Part model, mm, in its own coordinate system. A direction names the side the tool comes from. Give positions to 0.01 mm unless a question says otherwise; leave off trailing zeros. Write each loop counter-clockwise with the first axis right and the second up, starting at its lowest first coordinate (ties: lowest second). Pieces come first, ordered by that corner, then holes. Notation, with made-up numbers: (12, 20.5) - (44, 20.5) arc R8 ccw to (44, 26.5) - close; hole circle Ø5 at (73.25, -12). An arc over 180 degrees is marked (long way). Answer in a Markdown table with one row per item. Add a question column.
1. Band-saw the part on B-B on x = -2. Write the cut outline in (y, z).
2. Pull direction Z, two halves, no side cores. Call faces 1 (the flat face through (0, 0, 290)), 2 (the cylindrical face through (11, 2, 262)), 3 (the flat face through (9, 4, 138)): released by +Z, released by -Z, zero draft, split by the parting line, or undercut.
3. Band-saw the part on A-A on z = 105. Write the cut outline in (x, y).
4. Which spindle directions (+Z, -Z, +X, -X, +Y, -Y) get a long thin tool onto all of the face, cutting with end or side? Do faces 4 (the flat face through (13, 0.5, 265)), 5 (the flat face through (16, 1, 147)). Say none if no direction does.
5. Probe line 1 along X through (y, z) = (-1.4, 152); line 2 along Z through (x, y) = (7, 2); line 3 along Z through (x, y) = (6.5, 0.3) (3 decimals). List the from-to ranges inside material, lowest first.
6. Drop flat-ended pins along their axis: pin 1 Ø5.5 at (x, z) = (11, 265) entering from +Y; pin 2 Ø1.8 at (x, z) = (11, 67.5) entering from +Y; pin 3 Ø0.8 at (y, z) = (3.5, 141) entering from -X. Give the stop position or say it passes through.
```python
from build123d import *

# Parameters (mm, degrees)
SKETCH1_W           = 32
SKETCH1_H           = 5
BOSS_EXTRUDE1_DEPTH = 290
SKETCH2_W           = 14
SKETCH2_H           = 280
BOSS_EXTRUDE2_DEPTH = 1.5
SKETCH3_R           = 3
CUT_EXTRUDE1_DEPTH  = 3.5
SKETCH4_R           = 1.75
CUT_EXTRUDE2_DEPTH  = 4
SKETCH5_R           = 0.785
CUT_EXTRUDE3_DEPTH  = 6
SKETCH6_R           = 1.23
CUT_EXTRUDE4_DEPTH  = 7.5
LPATTERN1_COUNT     = 2
LPATTERN1_PITCH     = 95
SKETCH7_R           = 1.23
CUT_EXTRUDE5_DEPTH  = 7.5
SKETCH8_R           = 1.23
CUT_EXTRUDE6_DEPTH  = 7.5
LPATTERN2_COUNT     = 3
LPATTERN2_PITCH     = 61.5
SKETCH9_R           = 1.5
CUT_EXTRUDE7_DEPTH  = 7.5
SKETCH10_R          = 0.785
CUT_EXTRUDE8_DEPTH  = 8


with BuildPart() as part:
    # Sketch1 → Boss-Extrude1 (new body)
    with BuildSketch(Plane.XY):
        Rectangle(SKETCH1_W, SKETCH1_H)
    extrude(amount=BOSS_EXTRUDE1_DEPTH)

    # Sketch2 → Boss-Extrude2 (add)
    with BuildSketch(Plane(origin=(0, 2.5, 0), x_dir=(1, 0, 0), z_dir=(0, 1, 0))):
        with Locations((9, -140)):
            Rectangle(SKETCH2_W, SKETCH2_H)
    extrude(amount=BOSS_EXTRUDE2_DEPTH)

    # Sketch3 → Cut-Extrude1 (cut)
    with BuildSketch(Plane(origin=(0, 4, 0), x_dir=(1, 0, 0), z_dir=(0, 1, 0))):
        with Locations((11, -10)):
            Circle(SKETCH3_R)
        with Locations((11, -145)):
            Circle(SKETCH3_R)
        with Locations((11, -265)):
            Circle(SKETCH3_R)
    extrude(amount=-CUT_EXTRUDE1_DEPTH, mode=Mode.SUBTRACT)

    # Sketch4 → Cut-Extrude2 (cut, through all)
    with BuildSketch(Plane(origin=(0, 0.5, 0), x_dir=(1, 0, 0), z_dir=(0, 1, 0))):
        with Locations((11, -10)):
            Circle(SKETCH4_R)
        with Locations((11, -145)):
            Circle(SKETCH4_R)
        with Locations((11, -265)):
            Circle(SKETCH4_R)
    extrude(amount=-CUT_EXTRUDE2_DEPTH, mode=Mode.SUBTRACT)

    # Sketch5 → Cut-Extrude3 (cut, through all)
    with BuildSketch(Plane(origin=(0, 2.5, 0), x_dir=(1, 0, 0), z_dir=(0, 1, 0))):
        with Locations((-11.5, -282.5)):
            Circle(SKETCH5_R)
        with Locations((6.5, -282.5)):
            Circle(SKETCH5_R)
        with Locations((-11.5, -287.5)):
            Circle(SKETCH5_R)
        with Locations((6.5, -287.5)):
            Circle(SKETCH5_R)
    extrude(amount=-CUT_EXTRUDE3_DEPTH, mode=Mode.SUBTRACT)

    # Sketch6 → Cut-Extrude4 (cut, through all)
    with BuildSketch(Plane(origin=(0, 4, 0), x_dir=(1, 0, 0), z_dir=(0, 1, 0))):
        with Locations((11, -20)):
            Circle(SKETCH6_R)
    cut_extrude4 = extrude(amount=-CUT_EXTRUDE4_DEPTH, mode=Mode.SUBTRACT)

    # LPattern1: Cut-Extrude4 ×2
    with Locations(*[(0, 0, i * LPATTERN1_PITCH) for i in range(1, LPATTERN1_COUNT)]):
        add(cut_extrude4, mode=Mode.SUBTRACT)

    # Sketch7 → Cut-Extrude5 (cut, through all)
    with BuildSketch(Plane.XZ.offset(2.5)):
        with Locations((-11, 10)):
            Circle(SKETCH7_R)
        with Locations((-11, 140)):
            Circle(SKETCH7_R)
        with Locations((-11, 152)):
            Circle(SKETCH7_R)
        with Locations((-11, 270)):
            Circle(SKETCH7_R)
    extrude(amount=-CUT_EXTRUDE5_DEPTH, mode=Mode.SUBTRACT)

    # Sketch8 → Cut-Extrude6 (cut, through all)
    with BuildSketch(Plane.XZ.offset(2.5)):
        with Locations((8.5, 133)):
            Circle(SKETCH8_R)
    cut_extrude6 = extrude(amount=-CUT_EXTRUDE6_DEPTH, mode=Mode.SUBTRACT)

    # LPattern2: Cut-Extrude6 ×3
    with Locations(*[(0, 0, i * LPATTERN2_PITCH) for i in range(1, LPATTERN2_COUNT)]):
        add(cut_extrude6, mode=Mode.SUBTRACT)

    # Sketch9 → Cut-Extrude7 (cut, through all)
    with BuildSketch(Plane.XZ.offset(2.5)):
        with Locations((11, 67.5)):
            Circle(SKETCH9_R)
    extrude(amount=-CUT_EXTRUDE7_DEPTH, mode=Mode.SUBTRACT)

    # Sketch10 → Cut-Extrude8 (cut)
    with BuildSketch(Plane.XY.offset(290)):
        with Locations((13, 0)):
            Circle(SKETCH10_R)
        with Locations((8, 0)):
            Circle(SKETCH10_R)
    extrude(amount=-CUT_EXTRUDE8_DEPTH, mode=Mode.SUBTRACT)


solid = part.part
```
Values:
| question | item | result |
|---|---|---|
| 1 | outline | (-2.5, 0) - (2.5, 0) - (2.5, 290) - (-2.5, 290) - close |
| 2 | face 1 | released by +Z |
| 2 | face 2 | undercut |
| 2 | face 3 | zero draft |
| 3 | outline | (-16, -2.5) - (16, -2.5) - (16, 4) - (2, 4) - (2, 2.5) - (-16, 2.5) - close |
| 4 | face 4 | +Y |
| 4 | face 5 | +Z, -Z, +X, +Y, -Y |
| 5 | line 1 | x = -16 to -12.23, -9.77 to 16 |
| 5 | line 2 | z = 0 to 281.89, 283.11 to 286.89, 288.11 to 290 |
| 5 | line 3 | z = 0 to 281.715, 283.285 to 286.715, 288.285 to 290 |
| 6 | pin 1 | stops at y = 0.5 |
| 6 | pin 2 | passes through |
| 6 | pin 3 | stops at x = 2 |
